from build123d import *

# Parameters (mm, degrees)
F0_R     = 1.5875
F1_DEPTH = 3.048


with BuildPart() as f1:
    # F0 (on Front) → F1 (new body)
    with BuildSketch(Plane.XZ):
        with BuildLine():
            ThreePointArc((3.175, 0), (-2.2450640303, -2.2450640303), (0, 3.175))
            Line((0, 3.175), (0, 7.9375))
            ThreePointArc((0, 7.9375), (-4.4245915599, 6.589908632), (-7.3468104853, 3.0047099599))
            ThreePointArc((-7.3468104853, 3.0047099599), (-6.589908632, -4.4245915599), (0, -7.9375))
            ThreePointArc((0, -7.9375), (5.6126600757, -5.6126600757), (7.9375, 0))
            Line((7.9375, 0), (3.175, 0))
        make_face()
        with BuildLine():
            ThreePointArc((-7.3468104853, 3.0047099599), (-4.4245915599, 6.589908632), (0, 7.9375))
            Line((0, 7.9375), (0, 47.625))
            ThreePointArc((0, 47.625), (-10.2932687392, 51.4142958971), (-15.6726173523, 60.9732055229))
            Line((-15.6726173523, 60.9732055229), (-7.3468104853, 3.0047099599))
        make_face()
        with BuildLine():
            Line((0, 47.625), (0, 7.9375))
            ThreePointArc((0, 7.9375), (5.6126600757, 5.6126600757), (7.9375, 0))
            Line((7.9375, 0), (36.5125, 0))
            ThreePointArc((36.5125, 0), (38.7576827175, 5.5318559458), (44.2230965871, 7.9342561776))
            Line((44.2230965871, 7.9342561776), (18.1474563207, 7.1885464806))
            ThreePointArc((18.1474563207, 7.1885464806), (12.0333180798, 9.7922381017), (10.0323453348, 16.129272468))
            Line((10.0323453348, 16.129272468), (15.7504882737, 61.515625))
            ThreePointArc((15.7504882737, 61.515625), (10.5003255158, 51.59375), (0, 47.625))
        make_face()
        with BuildLine():
            Line((36.5125, 0), (7.9375, 0))
            ThreePointArc((7.9375, 0), (5.6126600757, -5.6126600757), (0, -7.9375))
            Line((0, -7.9375), (44.45, -7.9375))
            ThreePointArc((44.45, -7.9375), (38.8373399243, -5.6126600757), (36.5125, 0))
        make_face()
        with BuildLine():
            ThreePointArc((-15.6726173523, 60.9732055229), (-10.2932687392, 51.4142958971), (0, 47.625))
            Line((0, 47.625), (0, 60.325))
            ThreePointArc((0, 60.325), (-3.175, 63.5), (0, 66.675))
            Line((0, 66.675), (0, 79.375))
            ThreePointArc((0, 79.375), (-10.4995761896, 75.4069108016), (-15.7502383805, 65.4863574599))
            ThreePointArc((-15.7502383805, 65.4863574599), (-15.875, 63.5), (-15.7502383805, 61.5136425401))
            Line((-15.7502383805, 61.5136425401), (-15.6726173523, 60.9732055229))
        make_face()
        with BuildLine():
            Line((0, 60.325), (0, 47.625))
            ThreePointArc((0, 47.625), (10.5003255158, 51.59375), (15.7504882737, 61.515625))
            ThreePointArc((15.7504882737, 61.515625), (15.8438414904, 62.5058612634), (15.875, 63.5))
            ThreePointArc((15.875, 63.5), (15.8419565013, 64.5237378624), (15.742963564, 65.5432139445))
            ThreePointArc((15.742963564, 65.5432139445), (10.4780628847, 75.425846854), (0, 79.375))
            Line((0, 79.375), (0, 66.675))
            ThreePointArc((0, 66.675), (2.2450640303, 65.7450640303), (3.175, 63.5))
            ThreePointArc((3.175, 63.5), (2.2450640303, 61.2549359697), (0, 60.325))
        make_face()
        with BuildLine():
            ThreePointArc((44.2230965871, 7.9342561776), (38.7576827175, 5.5318559458), (36.5125, 0))
            ThreePointArc((36.5125, 0), (38.8373399243, -5.6126600757), (44.45, -7.9375))
            ThreePointArc((44.45, -7.9375), (50.0626600757, -5.6126600757), (52.3875, 0))
            ThreePointArc((52.3875, 0), (49.9818559458, 5.6923172825), (44.2230965871, 7.9342561776))
        make_face()
        with BuildLine():
            ThreePointArc((47.625, 0), (44.45, -3.175), (41.275, 0))
            ThreePointArc((41.275, 0), (44.45, 3.175), (47.625, 0))
        make_face(mode=Mode.SUBTRACT)
        with BuildLine():
            ThreePointArc((-15.7502383805, 61.5136425401), (-15.7137514185, 61.243090308), (-15.6726173523, 60.9732055229))
            Line((-15.6726173523, 60.9732055229), (-15.7502383805, 61.5136425401))
        make_face()
        with BuildLine():
            ThreePointArc((-15.7502383805, 65.4863574599), (-10.4995761896, 75.4069108016), (0, 79.375))
            Line((0, 79.375), (0, 104.775))
            ThreePointArc((0, 104.775), (-7.0279952587, 107.8709325992), (-9.4873396767, 115.1461742481))
            Line((-9.4873396767, 115.1461742481), (-15.7502383805, 65.4863574599))
        make_face()
        with Locations((-5.4959040135, 100.0252)):
            Circle(F0_R, mode=Mode.SUBTRACT)
        with BuildLine():
            Line((0, 104.775), (0, 79.375))
            ThreePointArc((0, 79.375), (10.4780628847, 75.425846854), (15.742963564, 65.5432139445))
            Line((15.742963564, 65.5432139445), (9.5016077683, 113.6328607214))
            ThreePointArc((9.5016077683, 113.6328607214), (6.4950413152, 107.3329300768), (0, 104.775))
        make_face()
        with BuildLine():
            ThreePointArc((-9.4873396767, 115.1461742481), (-7.0279952587, 107.8709325992), (0, 104.775))
            ThreePointArc((0, 104.775), (6.4950413152, 107.3329300768), (9.5016077683, 113.6328607214))
            ThreePointArc((9.5016077683, 113.6328607214), (9.5191501457, 113.9662253704), (9.525, 114.3))
            ThreePointArc((9.525, 114.3), (0.4235059498, 123.8155802614), (-9.4873396767, 115.1461742481))
        make_face()
        with BuildLine():
            ThreePointArc((3.175, 114.3), (2.2450640303, 112.0549359697), (0, 111.125))
            ThreePointArc((0, 111.125), (-2.2450640303, 116.5450640303), (3.175, 114.3))
        make_face(mode=Mode.SUBTRACT)
        with BuildLine():
            Line((0, 7.9375), (0, 3.175))
            ThreePointArc((0, 3.175), (2.2450640303, 2.2450640303), (3.175, 0))
            Line((3.175, 0), (7.9375, 0))
            ThreePointArc((7.9375, 0), (5.6126600757, 5.6126600757), (0, 7.9375))
        make_face()
    extrude(amount=F1_DEPTH)


solid = f1.part
Part model, mm, in its own coordinate system. A direction names the side the tool comes from. Coordinates: 2 decimals unless noted, no trailing zeros. Loops run counter-clockwise (first coordinate to the right, second up) from the corner with the lowest first, then second, coordinate; pieces in that order, holes last. Notation, with made-up numbers: M 20,44 L 37,44 A4 ccw 37,48 Z; hole C -14,82 d1. An arc over 180 degrees is marked long. Use a Markdown table: item, result. Add a question column.
Q1. Cut at B-B (z = 26.5). Write the cut outline in (x, y).
Q2. Pin check, flat tip, straight feed: P1, Ø8.5, axis at x = 0, z = 114.3, coming from the -Y side. Stop position of the tip, or through.
Q3. Probe L1, parallel to X at y = -1.05, z = -2; L2, parallel to Z at x = 17.5, y = -2.25; L3, parallel to X at y = -2.3, z = 114.3 (3 decimals). List the from-to ranges inside material, lowest first.
Q4. Cut at A-A (y = -1.55). Give the number of separate pieces and of enclosed holes in the cut face, and give its area (3 significant figures).
Q5. Which spindle directions (+Z, -Z, +X, -X, +Y, -Y) get a long thin tool onto all of the face, cutting with end or side? Do faces 1 (the cylindrical face through (12.1, -1.5, 9.72)), 2 (the flat face through (12.85, -1.5, 38.5)), 3 (the flat face through (3, -3.048, 59)). Say none if no direction does.
Q6. Cut at C-C (x = 27). Write the cut outline in (y, z).
Q7. Mould opens along Z. For faces 4 (the flat face through (3, 0, 59)), 5 (the cylindrical face through (-6.65, -1.503, -4.334)), 6 (the flat face through (-12.575, -1.503, 90.664)) say: +Z half, -Z half, draft (parallel to the pull), parting line (faces both ways), or undercut.
Worked out:
| question | item | result |
|---|---|---|
| 1 | outline | M -10.72,-3.05 L 11.34,-3.05 L 11.34,0 L -10.72,0 Z |
| 2 | P1 | stops at y = -3.05 |
| 3 | L1 | x = -7.68 to -2.47, 2.47 to 41.98, 46.92 to 52.13 |
| 3 | L2 | z = -7.94 to 7.2 |
| 3 | L3 | x = -9.594 to -3.175, 3.175 to 9.525 |
| 4 | separate pieces | 1 |
| 4 | enclosed holes | 5 |
| 4 | area | 3,580 mm2 |
| 5 | face 1 | +Y, -Y |
| 5 | face 2 | +X, +Y, -Y |
| 5 | face 3 | +Z, -Z, +X, -X, -Y |
| 6 | outline | M -3.05,-7.94 L 0,-7.94 L 0,7.44 L -3.05,7.44 Z |
| 7 | face 4 | draft |
| 7 | face 5 | undercut |
| 7 | face 6 | +Z half |
